Source: CAD feature listing. Evaluate the final solid. Frame: model axes, mm. Face numbers are marked on the shaded views. A direction names the side the tool comes from. Round coordinates to 2 decimals unless told otherwise and drop trailing zeros. Write each loop counter-clockwise with the first axis right and the second up, starting at its lowest first coordinate (ties: lowest second). Pieces come first, ordered by that corner, then holes.
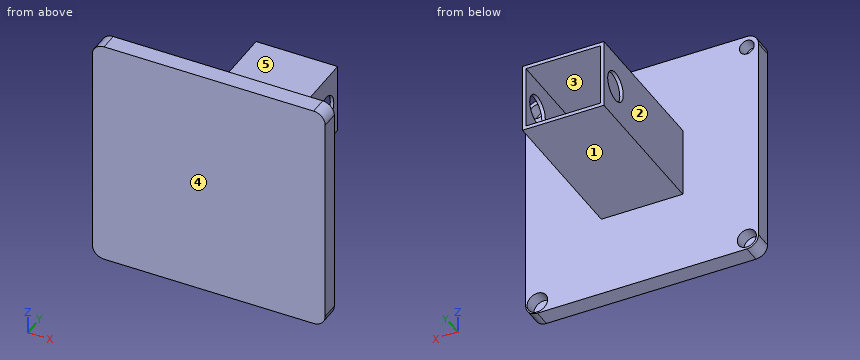
```python
from build123d import *

# Parameters (mm, degrees)
SALIENTE_EXTRUIR1_DEPTH = 15
CROQUIS2_W              = 70
CROQUIS2_H              = 60
CROQUIS2_W_2            = 64
CROQUIS2_H_2            = 54
SALIENTE_EXTRUIR2_DEPTH = 130
CROQUIS3_R              = 12.804907533
CORTAR_EXTRUIR1_DEPTH   = 88
CROQUIS4_R              = 8.190031249
CROQUIS4_R_2            = 8.81355523
CROQUIS4_R_3            = 6.340285024
CROQUIS4_R_4            = 6.633362886
CORTAR_EXTRUIR2_DEPTH   = 11


with BuildPart() as part:
    # Croquis1 → Saliente-Extruir1 (new body)
    with BuildSketch(Plane(origin=(0, 0, 0), x_dir=(1, 0, 0), z_dir=(0, 1, 0))):
        with BuildLine():
            Line((-90, 100), (90, 100))
            ThreePointArc((90, 100), (97.071067812, 97.071067812), (100, 90))
            Line((100, 90), (100, -90))
            ThreePointArc((100, -90), (97.071067812, -97.071067812), (90, -100))
            Line((90, -100), (-90, -100))
            ThreePointArc((-90, -100), (-97.071067812, -97.071067812), (-100, -90))
            Line((-100, -90), (-100, 90))
            ThreePointArc((-100, 90), (-97.071067812, 97.071067812), (-90, 100))
        make_face()
    extrude(amount=SALIENTE_EXTRUIR1_DEPTH)

    # Croquis2 → Saliente-Extruir2 (add)
    with BuildSketch(Plane(origin=(0, 15, 0), x_dir=(1, 0, 0), z_dir=(0, 1, 0))):
        Rectangle(CROQUIS2_W, CROQUIS2_H)
        Rectangle(CROQUIS2_W_2, CROQUIS2_H_2, mode=Mode.SUBTRACT)
    extrude(amount=SALIENTE_EXTRUIR2_DEPTH)

    # Croquis3 → Cortar-Extruir1 (cut)
    with BuildSketch(Plane(origin=(35, 0, 0), x_dir=(0, 0, -1), z_dir=(1, 0, 0))):
        with Locations((0, 125.915041201)):
            Circle(CROQUIS3_R)
    extrude(amount=-CORTAR_EXTRUIR1_DEPTH, mode=Mode.SUBTRACT)

    # Croquis4 → Cortar-Extruir2 (cut)
    with BuildSketch(Plane(origin=(0, 15, 0), x_dir=(1, 0, 0), z_dir=(0, 1, 0))):
        with Locations((-90, 90)):
            Circle(CROQUIS4_R)
        with Locations((90, 90)):
            Circle(CROQUIS4_R_2)
        with Locations((-90, -90)):
            Circle(CROQUIS4_R_3)
        with Locations((90, -90)):
            Circle(CROQUIS4_R_4)
    extrude(amount=-CORTAR_EXTRUIR2_DEPTH, mode=Mode.SUBTRACT)


solid = part.part
```
Q1. Mould query, pull axis X, two halves, no side actions, for the marked faces 1, 2 and 3. Classes: pulls with the +X half, pulls with the -X half, needs draft (parallel to the pull), parting line crosses it, or undercut.
Q2. Section query C-C, the plane x = 18.5. Output: boundary loops of the cut face in (y, z), and give its area (3 significant figures).
Q3. Pin query (flat end, axial travel): P1, Ø15.5, axis at y = 125.92, z = 0, coming from the +X side; P2, Ø14.5, axis at x = 90, z = 91, coming from the +Y side; P3, Ø10.5, axis at x = 90, z = -90, coming from the -Y side; P4, Ø6, axis at x = -28, y = 39, coming from the +Z side. Return the tip coordinate at first contact, or that it passes through.
Q4. Section query B-B, the plane y = 100. Output: boundary loops of the cut face in (x, z).
Q5. Section query A-A, the plane z = 0. Output: boundary loops of the cut face in (x, y), and give its area (3 significant figures).
Q6. Line query: line 1 (X direction, y = 10, z = -90); line 2 (Z direction, x = -90, y = 11.5); line 3 (Z direction, x = 90, y = 7.5). Output: solid intervals per line, ascending.
Q7. Set-up query: the marked faces 4 and 5. Return all of +Z, -Z, +X, -X, +Y, -Y with unobstructed straight access to the full face (end or side cutting, diameter ignored); none if empty.
Q8. Section query D-D, the plane y = 120. Output: boundary loops of the cut face in (x, z).
Filled in:
1. face 1: needs draft
1. face 2: pulls with the -X half
1. face 3: undercut
2. outline: (0, -100) - (15, -100) - (15, -30) - (145, -30) - (145, -27) - (15, -27) - (15, 27) - (145, 27) - (145, 30) - (15, 30) - (15, 100) - (0, 100) - close
2. area: 3,780 mm2
3. P1: passes through
3. P2: stops at y = 15
3. P3: stops at y = 0
3. P4: stops at z = 30
4. outline: (-35, -30) - (35, -30) - (35, 30) - (-35, 30) - close; hole (-32, -27) - (32, -27) - (32, 27) - (-32, 27) - close
5. outline: (-100, 0) - (100, 0) - (100, 15) - (35, 15) - (35, 113.11) - (32, 113.11) - (32, 15) - (-32, 15) - (-32, 113.11) - (-35, 113.11) - (-35, 15) - (-100, 15) - close; (-35, 138.72) - (-32, 138.72) - (-32, 145) - (-35, 145) - close; (32, 138.72) - (35, 138.72) - (35, 145) - (32, 145) - close
5. area: 3,630 mm2
6. line 1: x = -100 to -98.19, -81.81 to 81.19, 98.81 to 100
6. line 2: z = -100 to -98.19, -81.81 to 83.66, 96.34 to 100
6. line 3: z = -100 to -98.81, -81.19 to 83.37, 96.63 to 100
7. face 4: +Z, -Z, +X, -X, -Y
7. face 5: +Z, +X, -X, +Y
8. outline: (-35, -30) - (35, -30) - (35, -11.36) - (32, -11.36) - (32, -27) - (-32, -27) - (-32, -11.36) - (-35, -11.36) - close; (-35, 11.36) - (-32, 11.36) - (-32, 27) - (32, 27) - (32, 11.36) - (35, 11.36) - (35, 30) - (-35, 30) - close
